Autodesk Inventor part; units mm, degrees
ref_plane "YZ Plane" through (0, 0, 0) normal (1, 0, 0) x (0, 1, 0)
ref_plane "XZ Plane" through (0, 0, 0) normal (0, 1, 0) x (-1, 0, 0)
ref_plane "XY Plane" through (0, 0, 0) normal (0, 0, 1) x (1, 0, 0)
sketch "Sketch1" plane through (0, 0, 0) normal (0, 0, 1) x (1, 0, 0)
  line L0 (0, 0) -> (45.72, 0)
  line L1 (45.72, 0) -> (45.72, 44.45)
  line L2 (45.72, 44.45) -> (0, 44.45)
  line L3 (0, 44.45) -> (0, 0)
  dimension "d0" = 45.72
  dimension "d1" = 44.45
extrude "Extrusion1" add sketch "Sketch1" along normal blind 3.1496
sketch "Sketch2" plane through (0, 0, 3.1496) normal (0, 0, 1) x (1, 0, 0)
  line L0 (45.72, 44.45) -> (0, 44.45)
  line L1 (0, 44.45) -> (0, 0)
  line L2 (15.24, 44.45) -> (30.48, 44.45)
  line L3 (30.48, 44.45) -> (30.48, 41.3004)
  line L4 (30.48, 41.3004) -> (15.24, 41.3004)
  line L5 (15.24, 41.3004) -> (15.24, 44.45)
  line L6 (0, 29.6333) -> (3.1496, 29.6333)
  line L7 (3.1496, 29.6333) -> (3.1496, 14.8167)
  line L8 (3.1496, 14.8167) -> (0, 14.8167)
  line L9 (0, 14.8167) -> (0, 29.6333)
  dimension "d4" = 15.24
  dimension "d5" = 3.1496
  dimension "d6" = 15.24
  dimension "d7" = 3.1496
  dimension "d8" = 14.8167
  dimension "d9" = 14.8167
extrude "Extrusion2" cut sketch "Sketch2" against normal blind 3.1496
sketch "Sketch3" plane through (0, 0, 3.1496) normal (0, 0, 1) x (1, 0, 0)
  line L0 (0, 0) -> (45.72, 0)
  line L1 (45.72, 0) -> (45.72, 44.45)
  line L2 (45.72, 44.45) -> (0, 0)
  line L3 (45.72, 0) -> (45.72, 44.45)
extrude "Extrusion3" cut sketch "Sketch3" against normal blind 3.1496
equation "\"d0\" = angleLength"
equation "\"d1\" = angleHeight"
equation "\"d2\" = thick"
equation "\"d4\" = 0.333333 * angleLength"
equation "\"d5\" = thick"
equation "\"d6\" = 0.333333 * angleLength"
equation "\"d7\" = thick"
equation "\"d8\" = 0.333333 * angleHeight"
equation "\"d9\" = 0.333333 * angleHeight"
equation "\"d10\" = thick"
equation "\"d12\" = thick"
equation "\"thick\" = 3.1496"
equation "\"angleLength\" = 45.72"
equation "\"angleHeight\" = 44.45"
properties part number "AngleSide"
Source: CAD feature listing. Evaluate the final solid. Frame: model axes, mm. A direction names the side the tool comes from. Coordinates: 2 decimals unless noted, no trailing zeros. Loops run counter-clockwise (first coordinate to the right, second up) from the corner with the lowest first, then second, coordinate; pieces in that order, holes last. Notation, with made-up numbers: M 1,44.25 L 22,44.25 A21 cw 22,63.25 Z; hole C 81.25,45.25 d3. An arc over 180 degrees is marked long. Use a Markdown table: item, result. Add a question column.
Q1. Section query C-C, the plane x = 24. Return loops of the section in (y, z).
Q2. First-contact query: pin 1 (1 mm diameter, centred on x = 13, z = 2, fed in from -Y); pin 2 (1.5 mm diameter, centred on x = 24.5, z = 1.5, fed in from +Y); pin 3 (0.9 mm diameter, centred on y = 22, z = 2.5, fed in from -X). Flat tips, straight axial feed; report the tip coordinate or a pass-through.
Q3. Section query A-A, the plane z = 1.1. Return loops of the section in (x, y).
Q4. Material intervals for L1, parallel to Y at x = 42, z = 2.25; L2, parallel to Y at x = 13.5, z = 2.1 (3 decimals); L3, parallel to X at y = 21, z = 1.8, sorted ascending.
Q5. Draft query along X for faces 1 (the flat face through (2, 29.633, 2)), 2 (the flat face through (23.18, 22.536, 1.597)), 3 (the flat face through (23, 41.3, 2)). Return one class per face: pulls with the +X half, pulls with the -X half, needs draft (parallel to the pull), parting line crosses it, or undercut.
Q6. Section query B-B, the plane y = 28. Return loops of the section in (x, z), and give its area (3 significant figures).
Q7. Access query for faces 4 (the flat face through (2, 14.817, 2)), 5 (the flat face through (38, 44.45, 2)), 6 (the flat face through (15.24, 43, 2)). Directions: +Z, -Z, +X, -X, +Y, -Y. A direction counts if a zero-diameter tool reaches every point of the face in a straight line with its end or side. Return the directions, or none.
Result:
| question | item | result |
|---|---|---|
| 1 | outline | M 23.33,0 L 41.3,0 L 41.3,3.15 L 23.33,3.15 Z |
| 2 | pin 1 | stops at y = 12.15 |
| 2 | pin 2 | stops at y = 41.3 |
| 2 | pin 3 | stops at x = 3.15 |
| 3 | outline | M 0,0 L 45.72,44.45 L 30.48,44.45 L 30.48,41.3 L 15.24,41.3 L 15.24,44.45 L 0,44.45 L 0,29.63 L 3.15,29.63 L 3.15,14.82 L 0,14.82 Z |
| 4 | L1 | y = 40.83 to 44.45 |
| 4 | L2 | y = 13.125 to 44.45 |
| 4 | L3 | x = 3.15 to 21.6 |
| 5 | face 1 | needs draft |
| 5 | face 2 | pulls with the +X half |
| 5 | face 3 | undercut |
| 6 | outline | M 3.15,0 L 28.8,0 L 28.8,3.15 L 3.15,3.15 Z |
| 6 | area | 80.8 mm2 |
| 7 | face 4 | +Z, -Z, -X |
| 7 | face 5 | +Z, -Z, +X, -X, +Y |
| 7 | face 6 | +Z, -Z, +Y |
